Input: part model. Units: mm. Frame: model coordinates. Give positions to 0.01 mm unless a question says otherwise; leave off trailing zeros. Write each loop counter-clockwise with the first axis right and the second up, starting at its lowest first coordinate (ties: lowest second). Pieces come first, ordered by that corner, then holes.
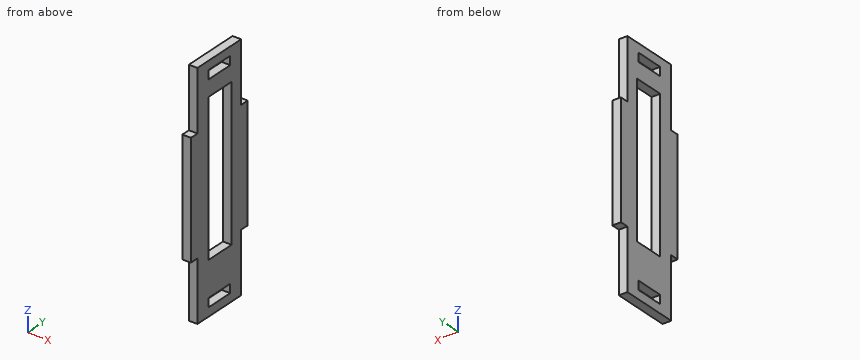
```python
from build123d import *

# Parameters (mm, degrees)
SKETCH1_W           = 3
SKETCH1_H           = 10
SKETCH1_W_2         = 52.177317389
SKETCH1_H_2         = 10.6108985
BOSS_EXTRUDE1_DEPTH = 3


with BuildPart() as part:
    # Sketch1 → Boss-Extrude1 (new body)
    with BuildSketch(Plane(origin=(0, 0, 0), x_dir=(0, 0, -1), z_dir=(1, 0, 0))):
        Polygon((-6, 0), (-6, 20), (15, 20), (15, 23), (55, 23), (55, 20), (76, 20), (76, 0), (55, 0), (55, -3), (15, -3), (15, 0), align=None)
        with Locations((-1.5, 10)):
            Rectangle(SKETCH1_W, SKETCH1_H, mode=Mode.SUBTRACT)
        with Locations((71.5, 10)):
            Rectangle(SKETCH1_W, SKETCH1_H, mode=Mode.SUBTRACT)
        with Locations((31.710045475, 10.30544925)):
            Rectangle(SKETCH1_W_2, SKETCH1_H_2, mode=Mode.SUBTRACT)
    extrude(amount=BOSS_EXTRUDE1_DEPTH)


solid = part.part
```
Item 1: Pin query (flat end, axial travel): pin 1 (1.5 mm diameter, centred on x = 1.5, z = -69.5, fed in from +Y); pin 2 (0.9 mm diameter, centred on x = 1.5, z = -9, fed in from -Y); pin 3 (1.5 mm diameter, centred on x = 1, y = -2, fed in from -Z). Return the tip coordinate at first contact, or that it passes through.
Item 2: Ray query, line 1 (Z direction, x = 1.8, y = 8.25); line 2 (Y direction, x = 0.2, z = -51); line 3 (Y direction, x = 0.5, z = -6.5). Return the intervals inside material, ascending.
Item 3: Section D-D (z = -58.5). Return loops of the section in (x, y), and give its area (3 significant figures).
Item 4: Section B-B (y = 6.5). Return loops of the section in (x, z), and give its area (3 significant figures).
Item 5: Section C-C (x = 1.35). Return loops of the section in (y, z), and give its area (3 significant figures).
Item 6: Section A-A (z = -17.5). Return loops of the section in (x, y), and give its area (3 significant figures).
Solved:
1. pin 1: stops at y = 20
1. pin 2: stops at y = 0
1. pin 3: stops at z = -55
2. line 1: z = -76 to -73, -70 to -57.8, -5.62 to 0, 3 to 6
2. line 2: y = -3 to 5, 15.61 to 23
2. line 3: y = 0 to 5, 15.61 to 20
3. outline: (0, 0) - (3, 0) - (3, 20) - (0, 20) - close
3. area: 60.0 mm2
4. outline: (0, -76) - (3, -76) - (3, -73) - (0, -73) - close; (0, -70) - (3, -70) - (3, -57.8) - (0, -57.8) - close; (0, -5.62) - (3, -5.62) - (3, 0) - (0, 0) - close; (0, 3) - (3, 3) - (3, 6) - (0, 6) - close
4. area: 71.5 mm2
5. outline: (-3, -55) - (0, -55) - (0, -76) - (20, -76) - (20, -55) - (23, -55) - (23, -15) - (20, -15) - (20, 6) - (0, 6) - (0, -15) - (-3, -15) - close; hole (5, -73) - (15, -73) - (15, -70) - (5, -70) - close; hole (5, -57.8) - (15.61, -57.8) - (15.61, -5.62) - (5, -5.62) - close; hole (5, 0) - (15, 0) - (15, 3) - (5, 3) - close
5. area: 1,270 mm2
6. outline: (0, -3) - (3, -3) - (3, 5) - (0, 5) - close; (0, 15.61) - (3, 15.61) - (3, 23) - (0, 23) - close
6. area: 46.2 mm2
